Geometry check sheet. Reference: the model listing, model coordinates, mm. Face numbers are marked on the shaded views. A direction names the side the tool comes from. Coordinates: 2 decimals unless noted, no trailing zeros. Order: outer loops, then holes, each group sorted by start corner. A loop starts at its lowest first (then second) coordinate and runs counter-clockwise, first axis right, second up. Notation, with made-up numbers: (55, -8) - (66, -8) arc R13 cw to (66, 4) - close; hole circle Ø10 at (11, 33.5). An arc over 180 degrees is marked (long way). Put each result on its own line as item: value.
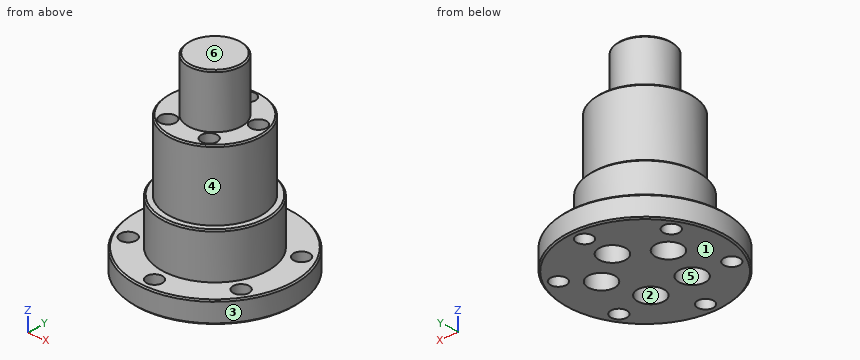
from build123d import *

# Parameters (mm, degrees)
SKETCH_2_R                   = 3
CUT_EXTRUDE_1_DEPTH          = 10
HOLE_WIZARD_M6_2_D           = 6
HOLE_WIZARD_M6_2_CBORE_D     = 10
HOLE_WIZARD_M6_2_CBORE_DEPTH = 6
PATTERN_CIRCULAR_1_COUNT     = 5
CHAMFER_1_SIZE               = 0.5


with BuildPart() as part:
    # 草图1 → 旋转1 (revolve)
    with BuildSketch(Plane(origin=(0, 0, 0), x_dir=(0, 0, -1), z_dir=(1, 0, 0)), mode=Mode.PRIVATE) as revolve_1_sk:
        Polygon((0, 0), (0, 10), (20, 10), (20, 17.5), (46, 17.5), (46, 20), (63, 20), (63, 30), (71, 30), (71, 0), align=None)
    revolve(revolve_1_sk.sketch.rotate(Axis((0, 0, 0), (0, 0, 1)), 90), axis=Axis((0, 0, 0), (0, 0, 1)))

    # 草图2 → 切除-拉伸1 (cut)
    with BuildSketch(Plane(origin=(0, 0, -71), x_dir=(-1, 0, 0), z_dir=(0, 0, -1))):
        with Locations((0, 25)):
            Circle(SKETCH_2_R)
        with Locations((21.650635095, 12.5)):
            Circle(SKETCH_2_R)
        with Locations((21.650635095, -12.5)):
            Circle(SKETCH_2_R)
        with Locations((0, -25)):
            Circle(SKETCH_2_R)
        with Locations((-21.650635095, -12.5)):
            Circle(SKETCH_2_R)
        with Locations((-21.650635095, 12.5)):
            Circle(SKETCH_2_R)
    extrude(amount=-CUT_EXTRUDE_1_DEPTH, mode=Mode.SUBTRACT)

    # M6 六角头螺栓的柱形沉头孔2 (through all)
    with Locations(Plane(origin=(0, 0, -71), x_dir=(-1, 0, 0), z_dir=(0, 0, -1))):
        with Locations((0, 13.5)):
            hole_wizard_m6_2 = CounterBoreHole(HOLE_WIZARD_M6_2_D / 2, HOLE_WIZARD_M6_2_CBORE_D / 2, HOLE_WIZARD_M6_2_CBORE_DEPTH)

    # 阵列(圆周)1: M6 六角头螺栓的柱形沉头孔2 ×5 about axis
    pattern_circular_1_axis = Axis((0, 0, 0), (0, 0, 1))
    for i in range(1, PATTERN_CIRCULAR_1_COUNT):
        add(hole_wizard_m6_2.rotate(pattern_circular_1_axis, i * 360 / PATTERN_CIRCULAR_1_COUNT), mode=Mode.SUBTRACT)

    # 倒角1
    chamfer_1_edges = [part.edges().sort_by_distance(p)[0] for p in [
        (17.5, 0, -20),
        (10, 0, 0),
        (30, 0, -71),
        (30, 0, -63),
        (20, 0, -46),
    ]]
    chamfer(chamfer_1_edges, length=CHAMFER_1_SIZE)


solid = part.part
Q1. Section check C-C on z = -10.5. Record the boundary of the cut face in (x, y), then the cut area to 3 significant figures.
Answer block:
outline: circle Ø20 at (0, 0)
area: 314 mm^2
Q2. Draft check along X on the marked faces 1, 2 and 3. Enter one of: pulls with the +X half, pulls with the -X half, needs draft (parallel to the pull), parting line crosses it, or undercut.
Answer block:
face 1: needs draft
face 2: undercut
face 3: parting line crosses it
Q3. Depth check by flat-ended pin: pin 1 Ø13 at (x, y) = (-7.94, -10.92) entering from -Z; pin 2 Ø3 at (x, z) = (3.5, -60) entering from -Y; pin 3 Ø8 at (x, y) = (12.84, 4.17) entering from -Z; pin 4 Ø5 at (x, y) = (-12.84, 4.17) entering from +Z. Enter the tip coordinate at first touch or a pass-through.
Answer block:
pin 1: stops at z = -71
pin 2: stops at y = -19.9
pin 3: stops at z = -65
pin 4: passes through
Q4. Access from +Z, -Z, +X, -X, +Y, -Y to the whole of each face (thin tool, end or side, straight path). Record for the marked faces 4, 5 and 6.
Answer block:
face 4: +Z
face 5: -Z
face 6: +Z, +X, -X, +Y, -Y
Q5. Thickness scan on L1, parallel to X at y = -13.5, z = -28; L2, parallel to Z at x = 5, y = -16; L3, parallel to Z at x = -4.5, y = 24. Record the ranges inside material, lowest first. Write a range as [from, to].
Answer block:
L1: x = [-11.14, -9.47], [-6.4, 6.4], [9.47, 11.14]
L2: z = [-71, -20]
L3: z = [-71, -63]
Q6. Section check A-A on z = -57.5. Record the boundary of the cut face in (x, y).
Answer block:
outline: circle Ø40 at (0, 0); hole circle Ø6 at (-12.84, 4.17); hole circle Ø6 at (-7.94, -10.92); hole circle Ø6 at (0, 13.5); hole circle Ø6 at (7.94, -10.92); hole circle Ø6 at (12.84, 4.17)
Q7. Section check B-B on x = 0.5. State how many separate pieces and enclosed holes the cut face has, then the cut area to 3 significant figures.
Answer block:
separate pieces: 4
enclosed holes: 0
area: 2,050 mm^2
